Check sheet for the modelled part. Datum: model origin and axes. Units: mm. A direction names the side the tool comes from. Coordinates: 2 decimals unless noted, no trailing zeros. Order: outer loops, then holes, each group sorted by start corner. A loop starts at its lowest first (then second) coordinate and runs counter-clockwise, first axis right, second up.
1. Draft check along Z on faces 1 (the flat face through (0, 0, 0)), 2 (the flat face through (20, -1, 3)), 3 (the cylindrical face through (-13.34, -1.48, 0.37)). Enter one of: released by +Z, released by -Z, zero draft, split by the parting line, or undercut.
2. Set-up check for faces 4 (the flat face through (-15, -3, -2)), 5 (the flat face through (0, -7, 4)), 6 (the flat face through (15, -3, -2)): record each of +Z, -Z, +X, -X, +Y, -Y from which the full face is reachable in a straight line by a thin tool's end or side.
3. Thickness scan on line 1 (X direction, y = -1.9, z = 0); line 2 (X direction, y = -18, z = -1); line 3 (Z direction, x = -15, y = -0.9). Record the ranges inside material, lowest first.
4. Cross-section at C-C (z = -3.5). Enter the section's corners in (x, y), then the cut area to 3 significant figures.
5. Cross-section at B-B (x = 15). Enter the section's corners in (y, z).
6. Cross-section at A-A (z = 0). Enter the section's corners in (x, y), then the cut area to 3 significant figures.
7. Gauge pin test, flat ends, axial feed: pin 1 Ø2.5 at (x, z) = (14.5, 1) entering from -Y; pin 2 Ø4 at (y, z) = (-13, 0.5) entering from -X; pin 3 Ø1 at (x, z) = (-8.5, -2.5) entering from -Y. Record the tip position at first contact, or that the pin passes through.
8. Cross-section at D-D (x = 0). Enter the section's corners in (y, z).
Autodesk Inventor part; units mm, degrees
ref_plane "YZ Plane" through (0, 0, 0) normal (1, 0, 0) x (0, 1, 0)
ref_plane "XZ Plane" through (0, 0, 0) normal (0, 1, 0) x (-1, 0, 0)
ref_plane "XY Plane" through (0, 0, 0) normal (0, 0, 1) x (1, 0, 0)
sketch "Sketch2" plane through (0, 0, 0) normal (0, 0, 1) x (1, 0, 0)
  line L0 (0, 0) -> (0, -18) construction
  line L1 (-9, 0) -> (-9, -18)
  line L2 (9, -18) -> (9, 0)
  arc A0 (9, 0) -> (-9, 0) centre (0, 0) ccw construction
  arc A1 (-9, -18) -> (9, -18) centre (0, -18) ccw
  arc A2 (6.5, -18) -> (-6.5, -18) centre (0, -18) ccw
  circle A3 centre (0, -18) radius 5 construction
  line L3 (-9, 0) -> (9, 0)
  line L4 (9, -18) -> (6.5, -18)
  arc A4 (-6.5, -18) -> (0, -24.5) centre (0, -18) ccw
  arc A5 (0, -24.5) -> (6.5, -18) centre (0, -18) ccw
  line L5 (-6.5, -18) -> (-9, -18)
  line L6 (6.5, -18) -> (-6.5, -18) construction
  line L7 (9, -18) -> (6.5, -18)
  line L8 (-9, -18) -> (-6.5, -18)
  point P0 (0, -9)
  dimension "d2" = 2.5
  dimension "d3" = 10
  dimension "d4" = 1.5
  dimension "d5" = 18
extrude "Extrusion1" add sketch "Sketch2" along normal mid plane 8 contours L3 L2 L4 A2 L5 L1 | L5 A4 A5 L4 A1
sketch "Sketch3" plane through (-9, 0, 4) normal (0, 1, 0) x (1, 0, 0)
  line L0 (-12, 0) -> (30, 0)
  line L1 (30, 0) -> (30, 8)
  line L2 (30, 8) -> (-12, 8)
  line L3 (-12, 8) -> (-12, 0)
  line L4 (-12, 0) -> (30, 8) construction
  line L5 (30, 0) -> (-12, 8) construction
  line L6 (0, 8) -> (18, 8)
  line L7 (0, 8) -> (0, 0)
  point P0 (9, 4)
  dimension "d8" = 12
extrude "Extrusion2" add sketch "Sketch3" against normal blind 3
sketch "Sketch4" plane through (-9, -3, 4) normal (0, -1, 0) x (1, 0, 0)
  line L0 (18, -8) -> (0, -8) construction
  line L1 (-12, 0) -> (0, 0) construction
  line L2 (-12, -8) -> (-12, 0) construction
  line L3 (0, 0) -> (18, 0) construction
  line L4 (30, 0) -> (30, -8) construction
  line L5 (30, -8) -> (18, -8) construction
  line L6 (0, -8) -> (0, 0) construction
  line L7 (0, -8) -> (-12, -8) construction
  line L8 (18, 0) -> (30, 0) construction
  line L9 (18, 0) -> (18, -8) construction
  line L10 (0, 0) -> (0, -8)
  line L11 (0, 0) -> (-12, 0)
  line L12 (-12, 0) -> (-12, -8)
  line L13 (-12, -8) -> (0, -8)
  line L14 (18, -8) -> (18, 0)
  line L15 (18, -8) -> (30, -8)
  line L16 (30, -8) -> (30, 0)
  line L17 (30, 0) -> (18, 0)
  point P0 (-6, -4)
  point P1 (24, -4)
  point P2 (24, 0)
  point P3 (-6, 0)
  point P4 (30, -4)
  point P5 (30, -4)
hole "Hole1" at (-15, -3, 0) at (15, -3, 0) direction (0, 1, 0) diameter 3.4 end through all
chamfer "Chamfer2" distance 1 angle 45 2 edges at (0, -11.5, -4) (0, -11.5, 4)
chamfer "Chamfer3" distance 2 angle 45 4 edges at (-21, -1.5, -4) (-21, -1.5, 4) (21, -1.5, -4) (21, -1.5, 4)
properties part number "driver gear stopper"
Data:
1. face 1: zero draft
1. face 2: released by +Z
1. face 3: undercut
2. face 4: +Z, -Z, -X, -Y
2. face 5: +Z, +X, -X, +Y, -Y
2. face 6: +Z, -Z, +X, -Y
3. line 1: x = -21 to -16.7, -13.3 to 13.3, 16.7 to 21
3. line 2: x = -9 to -6.5, 6.5 to 9
3. line 3: z = -4 to -1.7, 1.7 to 4
4. outline: (-19.5, -3) - (-9, -3) - (-9, -18) arc R9 ccw to (9, -18) - (9, -3) - (19.5, -3) - (19.5, 0) - (-19.5, 0) - close; hole circle Ø14 at (0, -18)
4. area: 360 mm2
5. outline: (-3, -4) - (0, -4) - (0, -1.7) - (-3, -1.7) - close; (-3, 1.7) - (0, 1.7) - (0, 4) - (-3, 4) - close
6. outline: (-21, -3) - (-16.7, -3) - (-16.7, 0) - (-21, 0) - close; (-13.3, -3) - (-9, -3) - (-9, -18) arc R9 ccw to (9, -18) - (9, -3) - (13.3, -3) - (13.3, 0) - (-13.3, 0) - close; (16.7, -3) - (21, -3) - (21, 0) - (16.7, 0) - close; hole circle Ø13 at (0, -18)
6. area: 370 mm2
7. pin 1: stops at y = -3
7. pin 2: stops at x = -9
7. pin 3: stops at y = -22.12
8. outline: (-27, -4) - (-25.5, -4) - (-24.5, -3) - (-24.5, 3) - (-25.5, 4) - (-27, 4) - close; (-11.5, -3) - (-10.5, -4) - (0, -4) - (0, 4) - (-10.5, 4) - (-11.5, 3) - close
